Geometry check sheet. Reference: the model listing, model coordinates, mm. A direction names the side the tool comes from. Give positions to 0.01 mm unless a question says otherwise; leave off trailing zeros. Write each loop counter-clockwise with the first axis right and the second up, starting at its lowest first coordinate (ties: lowest second). Pieces come first, ordered by that corner, then holes. Notation, with made-up numbers: M 81.25,59 L 108.25,59 A9 cw 108.25,76 Z; hole C -3,55.5 d1. An arc over 180 degrees is marked long. One line per item, written item: value. Start each with the question number.
1. Cross-section at B-B on y = 0. Record the cut outline in (x, z) (3 decimals), then the cut area to 3 significant figures.
2. Release check for a two-part mould opening along X. For faces 4 (the face through (3.6, 15.02, 1.33)), 5 (the face through (0, 0, 1.9)), 6 (the face through (8.072, 15.365, -1.139)) record: pulls with the +X half, pulls with the -X half, needs draft (parallel to the pull), parting line crosses it, or undercut.
3. Tool access check on faces 1 (the face through (-2.575, 19.877, 0.027)), 2 (the face through (-3.08, 17.3, 1.33)), 3 (the face through (4.98, 15.96, -1.32)). Record the directions out of +Z, -Z, +X, -X, +Y, -Y that give a thin tool (end or side, any length) a straight path to the whole face; none if there is none.
4. Cross-section at C-C on y = 20. Record the cut outline in (x, z), then the cut area to 3 significant figures.
5. Gauge pin test, flat end, axial feed: pin 1 (0.7 mm diameter, centred on x = 0.5, z = -0.5, fed in from +Y). Record the tip position at first contact, or that the pin passes through.
6. Scan lines: line 1 (X direction, y = 8, z = 0.9); line 2 (X direction, y = -1.5, z = 1); line 3 (Y direction, x = -0.5, z = 1.3). Record each from-to range of solid material in increasing order.
7. Cross-section at A-A on x = 0. Record the cut outline in (y, z) (3 decimals), then the cut area to 3 significant figures.
from build123d import *

# Parameters (mm, degrees)
ESBO_O1_R                  = 12.75
RESSALTO_EXTRUS_O1_DEPTH   = 1.9
ESBO_O1_R_2                = 12.25
RESSALTO_EXTRUS_O1_2_DEPTH = 1.9
ESBO_O1_3_R                = 12.75
ESBO_O1_3_R_2              = 12.25
RESSALTO_EXTRUS_O2_DEPTH   = 0.75
CHANFRO1_SIZE              = 1.5
ESBO_O1_4_R                = 12.75
ESBO_O1_4_R_2              = 12.25
RESSALTO_EXTRUS_O3_DEPTH   = 1.9


with BuildPart() as part:
    # Esbo_o1 → Ressalto-extrus_o1 (new body, symmetric)
    with BuildSketch(Plane.XY):
        with BuildLine():
            ThreePointArc((13.969531124, 7.695660998), (14.476708195, 6.827634982), (14.894166908, 5.913071715))
            ThreePointArc((14.894166908, 5.913071715), (0, -16.025), (-14.894166908, 5.913071715))
            ThreePointArc((-14.894166908, 5.913071715), (-14.476708195, 6.827634982), (-13.969531124, 7.695660998))
            Line((-13.969531124, 7.695660998), (-3.557120859, 23.620523756))
            ThreePointArc((-3.557120859, 23.620523756), (0, 25.544713963), (3.557120859, 23.620523756))
            Line((3.557120859, 23.620523756), (13.969531124, 7.695660998))
        make_face()
        Circle(ESBO_O1_R, mode=Mode.SUBTRACT)
        with BuildLine():
            ThreePointArc((-1.125, 21.294713963), (-2.575, 19.844713963), (-1.125, 18.394713963))
            Line((-1.125, 18.394713963), (1.125, 18.394713963))
            ThreePointArc((1.125, 18.394713963), (2.575, 19.844713963), (1.125, 21.294713963))
            Line((1.125, 21.294713963), (-1.125, 21.294713963))
        make_face(mode=Mode.SUBTRACT)
        with BuildLine():
            ThreePointArc((-5.72261878, 14.826624148), (-5.48070237, 13.670801302), (-4.324879525, 13.912717712))
            Line((-4.324879525, 13.912717712), (-2.858251232, 16.155796277))
            ThreePointArc((-2.858251232, 16.155796277), (-3.100167641, 17.311619123), (-4.255990487, 17.069702714))
            Line((-4.255990487, 17.069702714), (-5.72261878, 14.826624148))
        make_face(mode=Mode.SUBTRACT)
        with BuildLine():
            Line((4.255990487, 17.069702714), (5.72261878, 14.826624148))
            ThreePointArc((5.72261878, 14.826624148), (5.48070237, 13.670801302), (4.324879525, 13.912717712))
            Line((4.324879525, 13.912717712), (2.858251232, 16.155796277))
            ThreePointArc((2.858251232, 16.155796277), (3.100167641, 17.311619123), (4.255990487, 17.069702714))
        make_face(mode=Mode.SUBTRACT)
    extrude(amount=RESSALTO_EXTRUS_O1_DEPTH, both=True)



with BuildPart() as body_2:
    # Esbo_o1 → Ressalto-extrus_o1 2 (new body, symmetric)
    with BuildSketch(Plane.XY):
        Circle(ESBO_O1_R_2)
    extrude(amount=RESSALTO_EXTRUS_O1_2_DEPTH, both=True)


with BuildPart() as part_1:
    add(part.part)

    add(body_2.part)  # Ressalto-extrus_o2 merges body 2
    # Esbo_o1_3 → Ressalto-extrus_o2 (add, symmetric)
    with BuildSketch(Plane.XY):
        with BuildLine():
            Line((-4.255990487, 17.069702714), (-5.72261878, 14.826624148))
            ThreePointArc((-5.72261878, 14.826624148), (-5.48070237, 13.670801302), (-4.324879525, 13.912717712))
            Line((-4.324879525, 13.912717712), (-2.858251232, 16.155796277))
            ThreePointArc((-2.858251232, 16.155796277), (-3.100167641, 17.311619123), (-4.255990487, 17.069702714))
        make_face()
        Circle(ESBO_O1_3_R)
        Circle(ESBO_O1_3_R_2, mode=Mode.SUBTRACT)
        with BuildLine():
            Line((2.858251232, 16.155796277), (4.324879525, 13.912717712))
            ThreePointArc((4.324879525, 13.912717712), (5.48070237, 13.670801302), (5.72261878, 14.826624148))
            Line((5.72261878, 14.826624148), (4.255990487, 17.069702714))
            ThreePointArc((4.255990487, 17.069702714), (3.100167641, 17.311619123), (2.858251232, 16.155796277))
        make_face()
    extrude(amount=RESSALTO_EXTRUS_O2_DEPTH, both=True)

    # Chanfro1
    chanfro1_edges = [part_1.edges().sort_by_distance(p)[0] for p in [
        (8.763325992, 15.658092377, 1.9),
        (0, 25.544713963, 1.9),
        (-8.763325992, 15.658092377, 1.9),
        (-14.476708195, 6.827634982, 1.9),
        (0, -16.025, -1.9),
        (-14.476708195, 6.827634982, -1.9),
        (-8.763325992, 15.658092377, -1.9),
        (0, -16.025, 1.9),
        (0, 25.544713963, -1.9),
        (8.763325992, 15.658092377, -1.9),
        (14.476708195, 6.827634982, -1.9),
        (14.476708195, 6.827634982, 1.9),
    ]]
    chamfer(chanfro1_edges, length=CHANFRO1_SIZE)

    # Esbo_o1_4 → Ressalto-extrus_o3 (add)
    with BuildSketch(Plane.XY):
        Circle(ESBO_O1_4_R)
        Circle(ESBO_O1_4_R_2, mode=Mode.SUBTRACT)
    extrude(amount=-RESSALTO_EXTRUS_O3_DEPTH)


solid = part_1.part
Report:
1. outline: M -16.025,-0.4 L -14.525,-1.9 L 14.525,-1.9 L 16.025,-0.4 L 16.025,0.4 L 14.525,1.9 L 12.75,1.9 L 12.75,0.75 L 12.25,0.75 L 12.25,1.9 L -12.25,1.9 L -12.25,0.75 L -12.75,0.75 L -12.75,1.9 L -14.525,1.9 L -16.025,0.4 Z
1. area: 116 mm^2
2. face 4: undercut
2. face 5: needs draft
2. face 6: pulls with the +X half
3. face 1: +Z, -Z
3. face 2: +Z
3. face 3: -Z
4. outline: M -5.92,-0.4 L -4.13,-1.9 L -2.57,-1.9 L -2.57,1.9 L -4.13,1.9 L -5.92,0.4 Z; M 2.57,-1.9 L 4.13,-1.9 L 5.92,-0.4 L 5.92,0.4 L 4.13,1.9 L 2.57,1.9 Z
4. area: 20.1 mm^2
5. pin 1: stops at y = 25.54
6. line 1: x = -13.17 to -9.93, -9.28 to 9.28, 9.93 to 13.17
6. line 2: x = -15.35 to -12.66, -12.16 to 12.16, 12.66 to 15.35
6. line 3: y = -15.12 to -12.74, -12.24 to 12.24, 12.74 to 18.39, 21.29 to 24.61
7. outline: M -16.025,-0.4 L -14.525,-1.9 L 18.395,-1.9 L 18.395,1.9 L 12.75,1.9 L 12.75,0.75 L 12.25,0.75 L 12.25,1.9 L -12.25,1.9 L -12.25,0.75 L -12.75,0.75 L -12.75,1.9 L -14.525,1.9 L -16.025,0.4 Z; M 21.295,-1.9 L 24.045,-1.9 L 25.545,-0.4 L 25.545,0.4 L 24.045,1.9 L 21.295,1.9 Z
7. area: 141 mm^2
